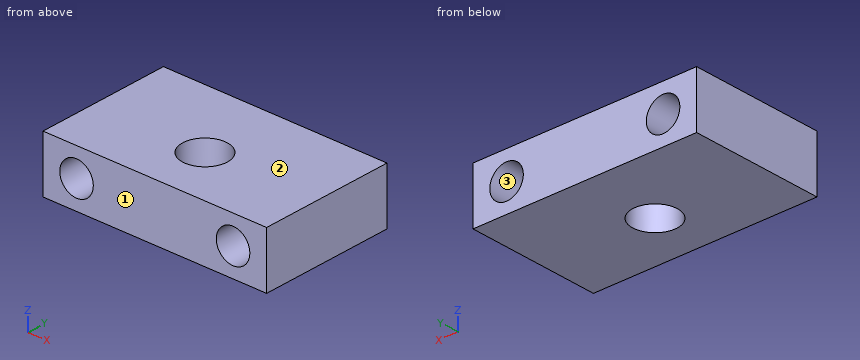
```python
from build123d import *

# Parameters (mm, degrees)
SKETCH_W     = 20
SKETCH_H     = 12
SKETCH_R     = 2
PAD_DEPTH    = 5
SKETCH001_R  = 1.5
POCKET_DEPTH = 12.001


with BuildPart() as part:
    # Sketch → Pad (new body)
    with BuildSketch(Plane.XY):
        with Locations((10, 6)):
            Rectangle(SKETCH_W, SKETCH_H)
        with Locations((10, 5)):
            Circle(SKETCH_R, mode=Mode.SUBTRACT)
    extrude(amount=PAD_DEPTH)

    # Sketch001 → Pocket (cut, through all)
    with BuildSketch(Plane.XZ):
        with Locations((3, 2.5)):
            Circle(SKETCH001_R)
        with Locations((17, 2.5)):
            Circle(SKETCH001_R)
    extrude(amount=-POCKET_DEPTH, mode=Mode.SUBTRACT)


solid = part.part
```
CAD build for the part. Positions are in the model's coordinates, mm. Face numbers are marked on the shaded views. Round coordinates to 2 decimals unless told otherwise and drop trailing zeros. Write each loop counter-clockwise with the first axis right and the second up, starting at its lowest first coordinate (ties: lowest second). Pieces come first, ordered by that corner, then holes. Notation, with made-up numbers: (26, 45.25) - (83, 45.25) arc R27 ccw to (83, 68.25) - close; hole circle Ø1 at (-34, -5). An arc over 180 degrees is marked (long way). Return JSON: item names as keys, results as strings. Group by question number.
Item 1: Probe probe 1 along Y at (x, z) = (10, 2.45); probe 2 along Z at (x, y) = (17, 8); probe 3 along X at (y, z) = (2.75, 1.25). List the from-to ranges inside material, lowest first.
Item 2: Band-saw the part on C-C on x = 10. List the corners of the cut face in (y, z), plus the area to 3 significant figures.
Item 3: Mould opens along Z. For the marked faces 1, 2 and 3 say: +Z half, -Z half, draft (parallel to the pull), parting line (faces both ways), or undercut.
Item 4: Band-saw the part on A-A on z = 2.5. List the corners of the cut face in (x, y), plus the area to 3 significant figures.
Item 5: Band-saw the part on D-D on z = 4.45. List the corners of the cut face in (x, y).
Item 6: Flat gauge pins, fed straight in: pin 1 Ø3.5 at (x, y) = (10, 5) entering from +Z; pin 2 Ø3 at (x, y) = (10, 3.5) entering from -Z. Where does each tip first touch, or does it go through?
Item 7: Band-saw the part on B-B on y = 5. List the corners of the cut face in (x, z).
Resolved:
{
 "1": {"probe 1": "y = 0 to 3, 7 to 12", "probe 2": "z = 0 to 1, 4 to 5", "probe 3": "x = 0 to 2.17, 3.83 to 16.17, 17.83 to 20"},
 "2": {"outline": "(0, 0) - (3, 0) - (3, 5) - (0, 5) - close; (7, 0) - (12, 0) - (12, 5) - (7, 5) - close", "area": "40.0 mm²"},
 "3": {"face 1": "draft", "face 2": "+Z half", "face 3": "undercut"},
 "4": {"outline": "(0, 0) - (1.5, 0) - (1.5, 12) - (0, 12) - close; (4.5, 0) - (15.5, 0) - (15.5, 12) - (4.5, 12) - close; (18.5, 0) - (20, 0) - (20, 12) - (18.5, 12) - close; hole circle Ø4 at (10, 5)", "area": "155 mm²"},
 "5": {"outline": "(0, 0) - (20, 0) - (20, 12) - (0, 12) - close; hole circle Ø4 at (10, 5)"},
 "6": {"pin 1": "passes through", "pin 2": "stops at z = 0"},
 "7": {"outline": "(0, 0) - (8, 0) - (8, 5) - (0, 5) - close; (12, 0) - (20, 0) - (20, 5) - (12, 5) - close; hole circle Ø3 at (3, 2.5); hole circle Ø3 at (17, 2.5)"}
}
